Read the model definition and answer for the solid it produces. Units are mm, in the model's axes. Coordinates: 2 decimals unless noted, no trailing zeros. Loops run counter-clockwise (first coordinate to the right, second up) from the corner with the lowest first, then second, coordinate; pieces in that order, holes last.
Q1. Flat-ended cylindrical pins translate along their axes: P1, Ø10, axis at x = 21.5, z = 20.5, coming from the -Y side; P2, Ø6, axis at y = 3, z = 31, coming from the +X side; P3, Ø8, axis at x = 16.5, z = 1, coming from the -Y side. Find the tip coordinate at first contact, or state that the pin passes through.
Q2. Straight lines are drawn through the part: line 1 (Y direction, x = 23.25, z = 19); line 2 (Z direction, x = 13.5, y = 12.5); line 3 (Z direction, x = 28.5, y = 6). For each, find the intervals that lie inside material, in ascending order.
Q3. Section A-A (x = 22.75) is taken. Give the vertices of the cut face in (y, z), then the cut area to 3 significant figures.
Q4. Section B-B (y = 5) is taken. Give the vertices of the cut face in (x, z).
Q5. Section C-C (z = 35) is taken. Give the vertices of the cut face in (x, y).
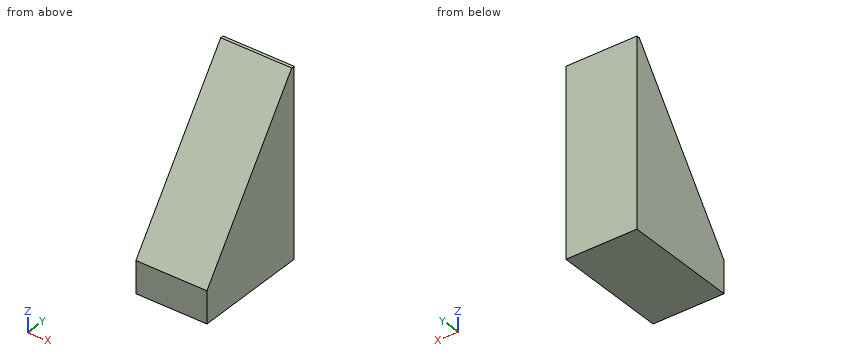
from build123d import *

# Parameters (mm, degrees)
BOX112015002004_W          = 23
BOX112015002004_H          = 34
BOX112015002004_DEPTH      = 80
BOX112015002004_ROLL_ANGLE = -36
BOX112015002003_W          = 21
BOX112015002003_H          = 34
BOX112015002003_DEPTH      = 55


with BuildPart() as cube074:
    # Box112015002004 → Box112015002004 (new body)
    with BuildSketch(Plane.XY):
        with Locations((11.5, 17)):
            Rectangle(BOX112015002004_W, BOX112015002004_H)
    extrude(amount=BOX112015002004_DEPTH)


with BuildPart() as cube074_1:
    # Box112015002004 roll: moved
    add(cube074.part.rotate(Axis((0, 0, 0), (1, 0, 0)), BOX112015002004_ROLL_ANGLE))


with BuildPart() as cube074_2:
    # Box112015002004 placement: moved
    add(cube074_1.part.moved(Location((10, -55, 0))))


with BuildPart() as cut130:
    # Box112015002003 → Box112015002003 (new body)
    with BuildSketch(Plane(origin=(11, -17, -15), x_dir=(1, 0, 0), z_dir=(0, 0, 1))):
        with Locations((10.5, 17)):
            Rectangle(BOX112015002003_W, BOX112015002003_H)
    extrude(amount=BOX112015002003_DEPTH)

    # Cut130: cut Cube074
    add(cube074_2.part, mode=Mode.SUBTRACT)


solid = cut130.part
Numbers:
1. P1: stops at y = -1.71
1. P2: passes through
1. P3: stops at y = -15.15
2. line 1: y = 0.83 to 17
2. line 2: z = -15 to 35.06
2. line 3: z = -15 to 26.12
3. outline: (-17, -15) - (17, -15) - (17, 40) - (16.09, 40) - (-17, -5.54) - close
3. area: 1,120 mm2
4. outline: (11, -15) - (32, -15) - (32, 24.74) - (11, 24.74) - close
5. outline: (11, 12.46) - (32, 12.46) - (32, 17) - (11, 17) - close
